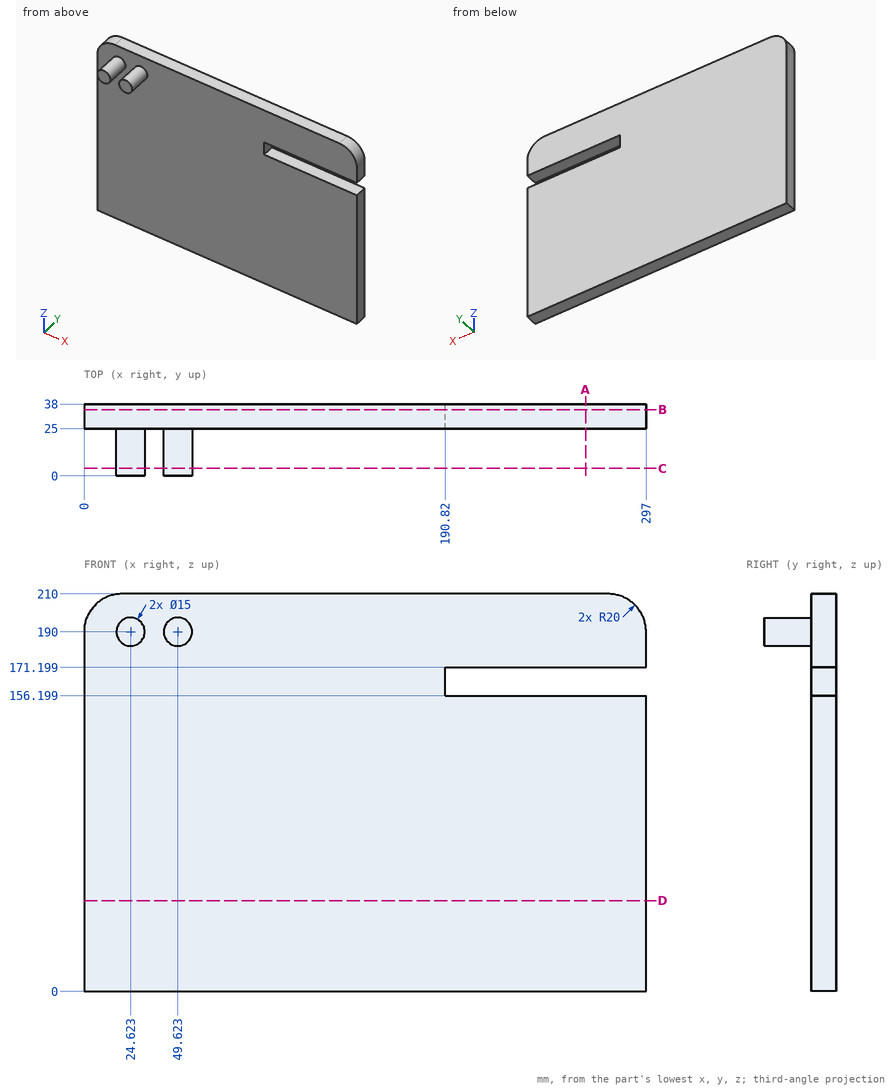
Input: dimensioned drawing with shaded views. Units: mm. Origin: part minimum x, y, z. Coordinates: 2 decimals unless noted, no trailing zeros. Loops run counter-clockwise (first coordinate to the right, second up) from the corner with the lowest first, then second, coordinate; pieces in that order, holes last.
Q1. Section A-A, the plane x = 265. Return the cut outline in (y, z), and give its area (4 significant figures).
Results are:
outline: (25, 0) - (38, 0) - (38, 156.2) - (25, 156.2) - close; (25, 171.2) - (38, 171.2) - (38, 210) - (25, 210) - close
area: 2,535 mm2
Q2. Section B-B, the plane y = 35. Return the cut outline in (x, z), and give its area (3 significant figures).
Results are:
outline: (0, 0) - (297, 0) - (297, 156.2) - (190.82, 156.2) - (190.82, 171.2) - (297, 171.2) - (297, 190) arc R20 ccw to (277, 210) - (20, 210) arc R20 ccw to (0, 190) - close
area: 60,600 mm2
Q3. Section C-C, the plane y = 4. Return the cut outline in (x, z), and give its area (3 significant figures).
Results are:
outline: circle Ø15 at (24.62, 190); circle Ø15 at (49.62, 190)
area: 353 mm2
Q4. Contact query for a flat-ended pin moving along its axis: pin 1 (6.5 mm diameter, centred on y = 32.5, z = 164, fed in from +X). Output: stop coordinate, or through.
Results are:
pin 1: stops at x = 190.82
Q5. Line query: line 1 along X through (y, z) = (3, 191); line 2 along Z through (x, y) = (264, 32); line 3 along X through (y, z) = (35.5, 168). Output: solid intervals per line, ascending.
Results are:
line 1: x = 17.19 to 32.06, 42.19 to 57.06
line 2: z = 0 to 156.2, 171.2 to 210
line 3: x = 0 to 190.82
Q6. Section D-D, the plane z = 48. Return the cut outline in (x, y).
Results are:
outline: (0, 25) - (297, 25) - (297, 38) - (0, 38) - close
